Input: part model. Units: mm. Frame: model coordinates. Round coordinates to 2 decimals unless told otherwise and drop trailing zeros. Write each loop counter-clockwise with the first axis right and the second up, starting at its lowest first coordinate (ties: lowest second). Pieces come first, ordered by that corner, then holes. Notation, with made-up numbers: (-5.75, 56) -> (11.25, 56) arc R18 cw to (11.25, 73) -> close; hole circle Ø7 at (-22.5, 7.5). An arc over 180 degrees is marked (long way). Write item = value, one per line. Start each with the question number.
```python
from build123d import *

# Parameters (mm, degrees)
SKETCH_2_R          = 4.55
CUT_EXTRUDE_1_DEPTH = 15
FILLET_1_R          = 1


with BuildPart() as part:
    # 스케치1 → 회전2 (revolve)
    with BuildSketch(Plane.XY):
        with BuildLine():
            Line((0, 12), (0, -12))
            ThreePointArc((0, -12), (-12, 0), (0, 12))
        make_face()
    revolve(axis=Axis((0, 11.789684906, 0), (0, -1, 0)))

    # 스케치2 → 컷-돌출1 (cut, symmetric)
    with BuildSketch(Plane.XY):
        with Locations(Location((0, 0, 0), (0, 0, 180))):
            Circle(SKETCH_2_R)
    extrude(amount=CUT_EXTRUDE_1_DEPTH, both=True, mode=Mode.SUBTRACT)

    # 필렛1
    fillet_1_edges = [part.edges().sort_by_distance(p)[0] for p in [
        (4.55, 0, 11.103940742),
        (4.55, 0, -11.103940742),
    ]]
    fillet(fillet_1_edges, radius=FILLET_1_R)


solid = part.part
```
1. Line query: line 1 along Y through (x, z) = (0, 5); line 2 along Y through (x, z) = (-1.5, -3.5); line 3 along Z through (x, y) = (3, -4.75). Output: solid intervals per line, ascending.
2. Section D-D (x = -6.5). Output: boundary loops of the cut face in (y, z).
3. Section A-A (z = 8.5). Output: boundary loops of the cut face in (x, y).
4. Section B-B (y = -8). Output: boundary loops of the cut face in (x, z), then the cut area to 3 significant figures.
5. Section C-C (z = -1.75). Output: boundary loops of the cut face in (x, y).
6. Pin query (flat end, axial travel): P1, Ø4, axis at x = -6, y = -7, coming from the -Z side; P2, Ø4, axis at x = 2, z = -2.5, coming from the -Y side; P3, Ø1.5, axis at x = -9, z = 0, coming from the +Y side; P4, Ø5.5, axis at x = 0, y = 0, coming from the -Z side. Return the tip coordinate at first contact, or that it passes through.
Check sheet entries:
q1.line_1 = -10.91 to -4.55, 4.55 to 10.91
q1.line_2 = -11.38 to -4.3, 4.3 to 11.38
q1.line_3 = -10.49 to 10.49
q2.outline = circle Ø20.17 at (0, 0)
q3.outline = circle Ø16.94 at (0, 0); hole circle Ø9.1 at (0, 0)
q4.outline = circle Ø17.89 at (0, 0)
q4.area = 251 mm2
q5.outline = circle Ø23.74 at (0, 0); hole circle Ø9.1 at (0, 0)
q6.P1 = -9.59
q6.P2 = -11.94
q6.P3 = 8.71
q6.P4 = through
